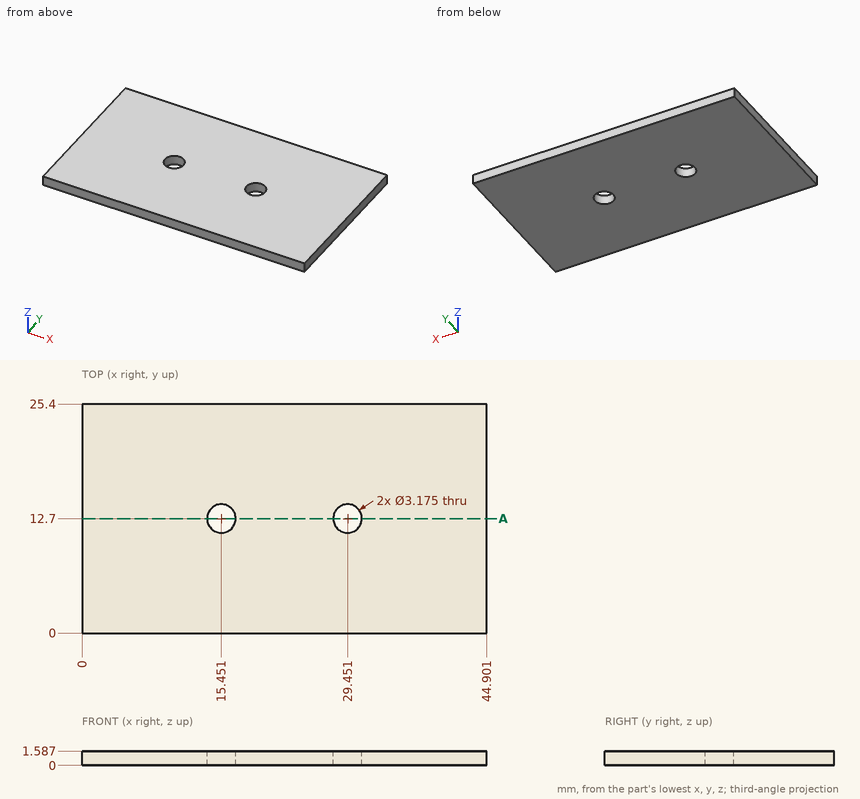
Design review of the part shown in the three views and the two pictorial views. Dimensions are in mm from the part's minimum x, y and z. Give positions to 0.01 mm unless a question says otherwise; leave off trailing zeros. Loops run counter-clockwise (first coordinate to the right, second up) from the corner with the lowest first, then second, coordinate; pieces in that order, holes last. Notation, with made-up numbers: M 11,76 L 25,76 A18 ccw 25,84 Z; hole C 89.25,-11.5 d6. An arc over 180 degrees is marked long. Answer as a JSON object with one key per item and string values. Group by question number.
Q1. Add section A-A on y = 12.7. Give the boundary of the cut face in (x, z).
Q2. Insertion check: P1, Ø3.5, axis at x = 29.45, y = 12.7, coming from the -Z side. The pin has a flat end and moves straight along its axis. Give the tip position at first contact, or say it passes through.
Q3. For probe 1 along X at (y, z) = (12.7, 0.7); probe 2 along X at (y, z) = (13.75, 0.7); probe 3 along Y at (x, z) = (29, 1.35), list the stretches that pass through material, from the lowest coordinate up. Write a range as [from, to].
Checked values:
{
 "1": {"outline": "M 0,0 L 13.86,0 L 13.86,1.59 L 0,1.59 Z; M 17.04,0 L 27.86,0 L 27.86,1.59 L 17.04,1.59 Z; M 31.04,0 L 44.9,0 L 44.9,1.59 L 31.04,1.59 Z"},
 "2": {"P1": "z = 0"},
 "3": {"probe 1": "[0, 13.86], [17.04, 27.86], [31.04, 44.9]", "probe 2": "[0, 14.26], [16.64, 28.26], [30.64, 44.9]", "probe 3": "[0, 11.18], [14.22, 25.4]"}
}
